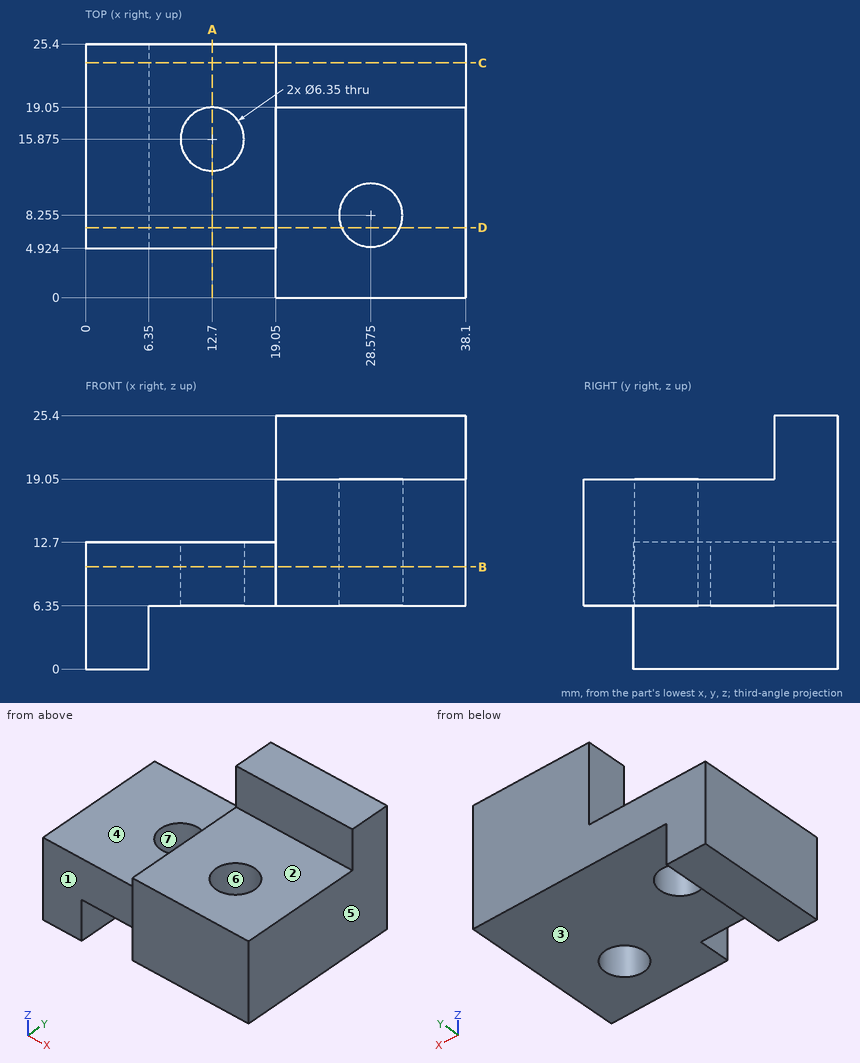
The drawing under review shows one solid part. Ordinate dimensions are in mm from its lowest x, y, z. A direction names the side the tool comes from. Give positions to 0.01 mm unless a question says otherwise; leave off trailing zeros. Write each loop counter-clockwise with the first axis right and the second up, starting at its lowest first coordinate (ties: lowest second). Pieces come first, ordered by that corner, then holes.
1. Add section C-C, the plane y = 23.5. Write out the cut boundary in (x, z), plus the area to 3 significant figures.
2. Add section D-D, the plane y = 7. Write out the cut boundary in (x, z).
3. For P1, Ø10, axis at x = 8, z = 5, coming from the -Y side; P2, Ø8, axis at x = 30.5, y = 11, coming from the +Z side; P3, Ø3, axis at y = 10, z = 14.5, coming from the -X side; P4, Ø8, axis at x = 30.5, y = 16.5, coming from the +Z side, all flat-tipped, find the tip position at first contact; note any pin that passes through.
4. Draft analysis for pull direction X (two halves, no side actions). For the marked faces 4, 5, 6 and 7, state which applies: +X half, -X half, draft (parallel to the pull), parting line (faces both ways), or undercut.
5. Tool access review of the marked faces 1, 2 and 3: name each direction out of +Z, -Z, +X, -X, +Y, -Y from which nothing blocks a thin tool from reaching the whole face with its end or side.
6. Add section B-B, the plane z = 10.25. Count the separate pieces of the cut face and the enclosed holes in it.
7. Add section A-A, the plane x = 12.7. Write out the cut boundary in (y, z).
8. Wall thickness on L1, parallel to Y at x = 12.7, z = 10.25; L2, parallel to X at y = 20.75, z = 15.25; L3, parallel to Y at x = 10.5, z = 12 (1 decimal): over which ranges is each line inside the solid? List them lowest first.
Worked answers:
1. outline: (0, 0) - (6.35, 0) - (6.35, 6.35) - (38.1, 6.35) - (38.1, 25.4) - (19.05, 25.4) - (19.05, 12.7) - (0, 12.7) - close
1. area: 524 mm2
2. outline: (0, 0) - (6.35, 0) - (6.35, 6.35) - (25.66, 6.35) - (25.66, 19.05) - (19.05, 19.05) - (19.05, 12.7) - (0, 12.7) - close; (31.49, 6.35) - (38.1, 6.35) - (38.1, 19.05) - (31.49, 19.05) - close
3. P1: stops at y = 4.92
3. P2: stops at z = 19.05
3. P3: stops at x = 19.05
3. P4: stops at z = 25.4
4. face 4: draft
4. face 5: +X half
4. face 6: undercut
4. face 7: undercut
5. face 1: +Z, -Z, -X, -Y
5. face 2: +Z, +X, -X, -Y
5. face 3: -Z, +X, +Y, -Y
6. separate pieces: 1
6. enclosed holes: 2
7. outline: (4.92, 6.35) - (12.7, 6.35) - (12.7, 12.7) - (4.92, 12.7) - close; (19.05, 6.35) - (25.4, 6.35) - (25.4, 12.7) - (19.05, 12.7) - close
8. L1: y = 4.92 to 12.7, 19.05 to 25.4
8. L2: x = 19.05 to 38.1
8. L3: y = 4.9 to 13.6, 18.2 to 25.4
